```python
from build123d import *

# Parameters (mm, degrees)
SKETCH1_W                     = 19.05
SKETCH1_H                     = 19.05
SKETCH1_W_2                   = 15.875
SKETCH1_H_2                   = 15.875
BOSS_EXTRUDE1_DEPTH           = 104.775
POWERSUPPLY_MOUNT_HOLES_REACH = 21.05
SKETCH4_R                     = 4.7625
CUT_EXTRUDE1_REACH            = 21.05
SKETCH5_R                     = 4.7625
SKETCH6_R                     = 4.7625
CUT_EXTRUDE2_DEPTH            = 20.05


with BuildPart() as part:
    # Sketch1 → Boss-Extrude1 (new body, symmetric)
    with BuildSketch(Plane(origin=(0, 0, 0), x_dir=(0, -1, 0), z_dir=(1, 0, 0))):
        Rectangle(SKETCH1_W, SKETCH1_H)
        Rectangle(SKETCH1_W_2, SKETCH1_H_2, mode=Mode.SUBTRACT)
    extrude(amount=BOSS_EXTRUDE1_DEPTH, both=True)

    # Sketch4 → PowerSupply Mount Holes (cut, up to next)
    with BuildSketch(Plane.XY.offset(-9.525), mode=Mode.PRIVATE) as powersupply_mount_holes_sk1:
        with Locations((-69.85, 0)):
            Circle(SKETCH4_R)
    powersupply_mount_holes_tool1 = extrude(powersupply_mount_holes_sk1.sketch, amount=POWERSUPPLY_MOUNT_HOLES_REACH, mode=Mode.PRIVATE) & part.part
    add(powersupply_mount_holes_tool1.solids().sort_by_distance((-69.85, 0, -9.525))[0], mode=Mode.SUBTRACT)
    # Sketch4 → PowerSupply Mount Holes (cut, up to next)
    with BuildSketch(Plane.XY.offset(-9.525), mode=Mode.PRIVATE) as powersupply_mount_holes_sk2:
        with Locations((69.85, 0)):
            Circle(SKETCH4_R)
    powersupply_mount_holes_tool2 = extrude(powersupply_mount_holes_sk2.sketch, amount=POWERSUPPLY_MOUNT_HOLES_REACH, mode=Mode.PRIVATE) & part.part
    add(powersupply_mount_holes_tool2.solids().sort_by_distance((69.85, 0, -9.525))[0], mode=Mode.SUBTRACT)

    # Sketch5 → Cut-Extrude1 (cut, up to next)
    with BuildSketch(Plane.XY.offset(9.525), mode=Mode.PRIVATE) as cut_extrude1_sk1:
        Circle(SKETCH5_R)
    cut_extrude1_tool1 = extrude(cut_extrude1_sk1.sketch, amount=-CUT_EXTRUDE1_REACH, mode=Mode.PRIVATE) & part.part
    add(cut_extrude1_tool1.solids().sort_by_distance((0, 0, 9.525))[0], mode=Mode.SUBTRACT)

    # Sketch6 → Cut-Extrude2 (cut, through all)
    with BuildSketch(Plane.XZ.offset(-9.525)):
        with Locations((-34.925, 0)):
            Circle(SKETCH6_R)
    extrude(amount=CUT_EXTRUDE2_DEPTH, mode=Mode.SUBTRACT)


solid = part.part
```
Input: part model. Units: mm. Frame: model coordinates. A direction names the side the tool comes from. Round coordinates to 2 decimals unless told otherwise and drop trailing zeros. Loops run counter-clockwise (first coordinate to the right, second up) from the corner with the lowest first, then second, coordinate; pieces in that order, holes last. Notation, with made-up numbers: M 10,21.25 L 69,21.25 A23 cw 69,34.25 Z; hole C -16,72.25 d10. An arc over 180 degrees is marked long. Answer in a Markdown table with one row per item. Add a question column.
1. Mould query, pull axis Z, two halves, no side actions, for faces 5 (the face through (74.25, -1.82, -8.74)), 6 (the face through (1, 0, -9.525)), 7 (the face through (1, -7.938, 0)). Classes: released by +Z, released by -Z, zero draft, split by the parting line, or undercut.
2. Ray query, probe 1 along X at (y, z) = (0, -8.7) (1 decimal); probe 2 along Z at (x, y) = (20, 4.5) (1 decimal). Return the intervals inside material, ascending.
3. Section B-B (x = 78.5). Output: boundary loops of the cut face in (y, z) (1 decimal), and give its area (3 significant figures).
4. Set-up query: faces 1 (the face through (1, -9.525, 0)), 2 (the face through (-65.45, -1.82, -8.74)), 3 (the face through (1, -5, 7.938)), 4 (the face through (-3.78, -2.9, 8.74)). Return all of +Z, -Z, +X, -X, +Y, -Y with unobstructed straight access to the full face (end or side cutting, diameter ignored); none if empty.
5. Section A-A (z = 0). Output: boundary loops of the cut face in (x, y) (1 decimal), and give its area (3 significant figures).
6. Contact query for flat-ended pins moving along their axis: pin 1 (10 mm diameter, centred on y = 0.5, z = 0.5, fed in from +X); pin 2 (5.5 mm diameter, centred on x = 0, y = 0, fed in from +Z). Output: stop coordinate, or through.
Values follow:
| question | item | result |
|---|---|---|
| 1 | face 5 | zero draft |
| 1 | face 6 | released by -Z |
| 1 | face 7 | undercut |
| 2 | probe 1 | -104.8 to -74.6, -65.1 to 65.1, 74.6 to 104.8 |
| 2 | probe 2 | -9.5 to -7.9, 7.9 to 9.5 |
| 3 | outline | M -9.5,-9.5 L 9.5,-9.5 L 9.5,9.5 L -9.5,9.5 Z; hole M -7.9,-7.9 L 7.9,-7.9 L 7.9,7.9 L -7.9,7.9 Z |
| 3 | area | 111 mm^2 |
| 4 | face 1 | +Z, -Z, +X, -X, -Y |
| 4 | face 2 | -Z |
| 4 | face 3 | +X, -X |
| 4 | face 4 | +Z |
| 5 | outline | M -104.8,-9.5 L -39.7,-9.5 L -39.7,-7.9 L -104.8,-7.9 Z; M -104.8,7.9 L -39.7,7.9 L -39.7,9.5 L -104.8,9.5 Z; M -30.2,-9.5 L 104.8,-9.5 L 104.8,-7.9 L -30.2,-7.9 Z; M -30.2,7.9 L 104.8,7.9 L 104.8,9.5 L -30.2,9.5 Z |
| 5 | area | 635 mm^2 |
| 6 | pin 1 | through |
| 6 | pin 2 | z = -7.94 |
